Input: part model. Units: mm. Frame: model coordinates. A direction names the side the tool comes from. Round coordinates to 2 decimals unless told otherwise and drop trailing zeros. Order: outer loops, then holes, each group sorted by start corner. A loop starts at its lowest first (then second) coordinate and runs counter-clockwise, first axis right, second up. Notation, with made-up numbers: M 62,-24 L 93,-24 A19 ccw 93,13 Z; hole C -1,45 d2. An arc over 180 degrees is marked long. One line per question, with ' | ' between items.
```python
from build123d import *

# Parameters (mm, degrees)
SKETCH1_R           = 9
SKETCH1_R_2         = 6
SKETCH1_R_3         = 4
BOSS_EXTRUDE1_DEPTH = 8
SKETCH3_R           = 4
BOSS_EXTRUDE2_DEPTH = 3
SKETCH4_R           = 6
BOSS_EXTRUDE3_DEPTH = 3


with BuildPart() as part:
    # Sketch1 → Boss-Extrude1 (new body)
    with BuildSketch(Plane(origin=(0, 0, 0), x_dir=(1, 0, 0), z_dir=(0, 1, 0))):
        with BuildLine():
            Line((82, 32.334641746), (22.899881176, 32.334641746))
            ThreePointArc((22.899881176, 32.334641746), (14.88590337, 33.106300041), (7.166404253, 35.392919854))
            Line((7.166404253, 35.392919854), (-45.003147253, 56.470786852))
            ThreePointArc((-45.003147253, 56.470786852), (-54.304086029, 53.978607818), (-54.472135955, 44.351033997))
            Line((-54.472135955, 44.351033997), (-14.562305899, -10.580134541))
            ThreePointArc((-14.562305899, -10.580134541), (-5.562305899, -17.119017293), (5.562305899, -17.119017293))
            Line((5.562305899, -17.119017293), (85.708203932, 8.92196355))
            ThreePointArc((85.708203932, 8.92196355), (93.852260087, 22.211855326), (82, 32.334641746))
        make_face()
        Circle(SKETCH1_R, mode=Mode.SUBTRACT)
        with Locations((82, 20.334641746)):
            Circle(SKETCH1_R_2, mode=Mode.SUBTRACT)
        with Locations((-48, 49.053316016)):
            Circle(SKETCH1_R_3, mode=Mode.SUBTRACT)
    extrude(amount=BOSS_EXTRUDE1_DEPTH)

    # Sketch3 → Boss-Extrude2 (add, symmetric)
    with BuildSketch(Plane(origin=(-19.984698578, 0, -27.506577809), x_dir=(0.809016994, 0, -0.587785252), z_dir=(0.587785252, 0, 0.809016994))):
        with BuildLine():
            Line((-18, 8), (11.512683232, 8))
            Line((11.512683232, 8), (-2.309906432, 56.205098847))
            ThreePointArc((-2.309906432, 56.205098847), (-11.113384808, 61.92214455), (-18, 54))
            Line((-18, 54), (-18, 8))
        make_face()
        with Locations((-10, 54)):
            Circle(SKETCH3_R, mode=Mode.SUBTRACT)
    extrude(amount=BOSS_EXTRUDE2_DEPTH, both=True)

    # Sketch4 → Boss-Extrude3 (add, symmetric)
    with BuildSketch(Plane(origin=(32.335921554, 0, -10.506577809), x_dir=(-0.309016994, 0, -0.951056516), z_dir=(0.951056516, 0, -0.309016994))):
        with BuildLine():
            Line((-18, 8), (-18, 56))
            ThreePointArc((-18, 56), (-7.254341559, 67.934262744), (5.737771209, 58.49494029))
            Line((5.737771209, 58.49494029), (16.470802099, 8))
            Line((16.470802099, 8), (-18, 8))
        make_face()
        with Locations((-6, 56)):
            Circle(SKETCH4_R, mode=Mode.SUBTRACT)
    extrude(amount=BOSS_EXTRUDE3_DEPTH, both=True)


solid = part.part
```
Item 1: Section query C-C, the plane z = -42. Return loops of the section in (x, y).
Report:
outline: M -52.76,0 L -9.19,0 L -9.19,8 L -52.76,8 Z
Item 2: Section query B-B, the plane y = 19. Return loops of the section in (x, z).
Report:
outline: M -36.31,-19.35 L -14.99,-34.85 L -11.46,-29.99 L -32.78,-14.5 Z; M 25.12,-23.02 L 30.82,-24.87 L 40.75,5.69 L 35.05,7.54 Z
Item 3: Mould query, pull axis Z, two halves, no side actions, for faces 6 (the flat face through (-18.553, 3.944, -45.784)), 7 (the cylindrical face through (93.887, 3.944, -21.977)), 8 (the flat face through (30.828, 31.753, -5.439)), 9 (the cylindrical face through (76.006, 3.944, -20.598)). Classes: +Z half, -Z half, draft (parallel to the pull), parting line (faces both ways), or undercut.
Report:
face 6: -Z half | face 7: parting line | face 8: +Z half | face 9: undercut
Item 4: Line query: line 1 along Y through (x, z) = (-3, -39); line 2 along Z through (x, y) = (82, 4.25); line 3 along X through (y, z) = (22, -21). Output: solid intervals per line, ascending. Write a range as from..to.
Report:
line 1: 0..8 | line 2: -32.33..-26.33, -14.33..-7.72 | line 3: -34.04..-23.84, 25.77..32.08
Item 5: Section query A-A, the plane x = -48. Return loops of the section in (y, z).
Report:
outline: M 0,-57.05 L 8,-57.05 L 8,-53.05 L 0,-53.05 Z; M 0,-45.05 L 8,-45.05 L 8,-35.44 L 0,-35.44 Z
Item 6: First-contact query: pin 1 (8 mm diameter, centred on x = 74.5, z = -40, fed in from +Y); pin 2 (3 mm diameter, centred on x = 56, z = -8.5, fed in from -Y); pin 3 (4 mm diameter, centred on y = 18, z = -21, fed in from +X); pin 4 (9 mm diameter, centred on x = -48, z = -49.05, fed in from +Y). Flat tips, straight axial feed; report the tip coordinate or a pass-through.
Report:
pin 1: through | pin 2: y = 0 | pin 3: x = 32.73 | pin 4: y = 8
Item 7: Access query for faces 1 (the flat face through (18, 8, -20)), 2 (the flat face through (28.97, 33.6, -21.01)), 3 (the flat face through (-27.19, 29.38, -25.98)), 4 (the flat face through (-23.7, 29.4, -21.1)), 5 (the flat face through (36.534, 31.753, -7.293)). Directions: +Z, -Z, +X, -X, +Y, -Y. A direction counts if a zero-diameter tool reaches every point of the face in a straight line with its end or side. Return the directions, or none.
Report:
face 1: +Y | face 2: -Z, +Y | face 3: -Z, -X, +Y | face 4: +Z, +Y | face 5: -Z, +X, +Y
Item 8: Section query D-D, the plane x = 72.5. Return loops of the section in (y, z).
Report:
outline: M 0,-32.33 L 8,-32.33 L 8,-4.63 L 0,-4.63 Z
